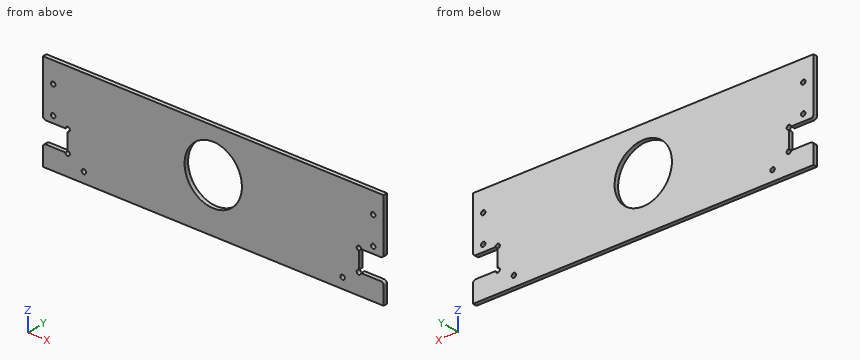
```python
from build123d import *

# Parameters (mm, degrees)
SKETCH_1_W          = 250
SKETCH_1_H          = 70
EXTRUDE_1_DEPTH     = 3
SKETCH_2_R          = 1.6
CUT_EXTRUDE_1_DEPTH = 130.842211934
SKETCH_4_W          = 18.1
SKETCH_4_H          = 15.2
CUT_EXTRUDE_3_DEPTH = 130.842211934
FILLET_2_R          = 2
SKETCH_5_R          = 1.6
CUT_EXTRUDE_4_DEPTH = 130.842211934
SKETCH_6_R          = 21.05
CUT_EXTRUDE_5_DEPTH = 130.842211934


with BuildPart() as part:
    # 草图1 → 凸台-拉伸1 (new body)
    with BuildSketch(Plane(origin=(0, 0, 0), x_dir=(1, 0, 0), z_dir=(0, 1, 0))):
        Rectangle(SKETCH_1_W, SKETCH_1_H)
    extrude(amount=EXTRUDE_1_DEPTH)

    # 草图2 → 切除-拉伸1 (cut, through all)
    with BuildSketch(Plane(origin=(0, 3, 0), x_dir=(1, 0, 0), z_dir=(0, 1, 0))):
        with Locations(Location((-95, 27.5, 0), (0, 0, 270))):
            Circle(SKETCH_2_R)
        with Locations(Location((95, 27.5, 0), (0, 0, 270))):
            Circle(SKETCH_2_R)
        with Locations(Location((-117.5, 0, 0), (0, 0, 270))):
            Circle(SKETCH_2_R)
        with Locations(Location((-117.5, -20, 0), (0, 0, 270))):
            Circle(SKETCH_2_R)
        with Locations(Location((117.5, -20, 0), (0, 0, 90))):
            Circle(SKETCH_2_R)
        with Locations(Location((117.5, 0, 0), (0, 0, 90))):
            Circle(SKETCH_2_R)
    extrude(amount=-CUT_EXTRUDE_1_DEPTH, mode=Mode.SUBTRACT)

    # 草图4 → 切除-拉伸3 (cut, through all)
    with BuildSketch(Plane(origin=(0, 3, 0), x_dir=(1, 0, 0), z_dir=(0, 1, 0))):
        with Locations((-115.95, 12.5)):
            Rectangle(SKETCH_4_W, SKETCH_4_H)
        with Locations((115.95, 12.5)):
            Rectangle(SKETCH_4_W, SKETCH_4_H)
    extrude(amount=-CUT_EXTRUDE_3_DEPTH, mode=Mode.SUBTRACT)

    # 圆角2
    fillet_2_edges = [part.edges().sort_by_distance(p)[0] for p in [
        (-125, 1.5, -4.9),
        (-125, 1.5, -20.1),
        (125, 1.5, -20.1),
        (125, 1.5, -4.9),
    ]]
    fillet(fillet_2_edges, radius=FILLET_2_R)

    # 草图5 → 切除-拉伸4 (cut, through all)
    with BuildSketch(Plane(origin=(0, 3, 0), x_dir=(1, 0, 0), z_dir=(0, 1, 0))):
        with Locations((-106.9, 20.1)):
            Circle(SKETCH_5_R)
        with Locations((-106.9, 4.9)):
            Circle(SKETCH_5_R)
        with Locations((106.9, 4.9)):
            Circle(SKETCH_5_R)
        with Locations((106.9, 20.1)):
            Circle(SKETCH_5_R)
    extrude(amount=-CUT_EXTRUDE_4_DEPTH, mode=Mode.SUBTRACT)

    # 草图6 → 切除-拉伸5 (cut, through all)
    with BuildSketch(Plane(origin=(0, 3, 0), x_dir=(1, 0, 0), z_dir=(0, 1, 0))):
        with Locations(Location((0, -3.75, 0), (0, 0, 270))):
            Circle(SKETCH_6_R)
    extrude(amount=-CUT_EXTRUDE_5_DEPTH, mode=Mode.SUBTRACT)


solid = part.part
```
Source: CAD feature listing. Evaluate the final solid. Frame: model axes, mm. Give positions to 0.01 mm unless a question says otherwise; leave off trailing zeros. Write each loop counter-clockwise with the first axis right and the second up, starting at its lowest first coordinate (ties: lowest second). Pieces come first, ordered by that corner, then holes. Notation, with made-up numbers: (1, 65) - (22, 65) arc R21 ccw to (22, 82) - close; hole circle Ø5 at (-34, -34). An arc over 180 degrees is marked (long way). One line per item, written item: value. Start each with the question number.
Q1. Material intervals for probe 1 along X at (y, z) = (0.9, -27.5); probe 2 along X at (y, z) = (1.8, 3.75); probe 3 along Z at (x, y) = (-95, 1.05), sorted ascending. Write a range as from..to.
Q2. Section query B-B, the plane x = 0. Return the cut outline in (y, z), then the cut area to 3 significant figures.
Q3. Section query C-C, the plane y = 0.7. Return the cut outline in (x, z).
Q4. Section query A-A, the plane z = 3.75. Return the cut outline in (x, y), then the cut area to 3 significant figures.
Q5. First-contact query: pin 1 Ø3 at (x, z) = (117.5, 0) entering from +Y; pin 2 Ø1.5 at (y, z) = (1, -14.5) entering from -X. Flat tips, straight axial feed; report the tip coordinate or a pass-through.
Answer:
1. probe 1: x = -125..-96.6, -93.4..93.4, 96.6..125
1. probe 2: x = -125..-21.05, 21.05..125
1. probe 3: z = -35..-29.1, -25.9..35
2. outline: (0, -35) - (3, -35) - (3, -17.3) - (0, -17.3) - close; (0, 24.8) - (3, 24.8) - (3, 35) - (0, 35) - close
2. area: 83.7 mm2
3. outline: (-125, -35) - (125, -35) - (125, -22.1) arc R2 ccw to (123, -20.1) - (108.5, -20.1) arc R1.6 cw (long way) to (106.9, -18.5) - (106.9, -6.5) arc R1.6 cw (long way) to (108.5, -4.9) - (123, -4.9) arc R2 ccw to (125, -2.9) - (125, 35) - (-125, 35) - (-125, -2.9) arc R2 ccw to (-123, -4.9) - (-108.5, -4.9) arc R1.6 cw (long way) to (-106.9, -6.5) - (-106.9, -18.5) arc R1.6 cw (long way) to (-108.5, -20.1) - (-123, -20.1) arc R2 ccw to (-125, -22.1) - close; hole circle Ø3.2 at (-117.5, 0); hole circle Ø3.2 at (-117.5, 20); hole circle Ø3.2 at (-95, -27.5); hole circle Ø42.1 at (0, 3.75); hole circle Ø3.2 at (95, -27.5); hole circle Ø3.2 at (117.5, 0); hole circle Ø3.2 at (117.5, 20)
4. outline: (-125, 0) - (-21.05, 0) - (-21.05, 3) - (-125, 3) - close; (21.05, 0) - (125, 0) - (125, 3) - (21.05, 3) - close
4. area: 624 mm2
5. pin 1: passes through
5. pin 2: stops at x = -106.9
